from build123d import *

# Parameters (mm, degrees)
SKETCH1_R           = 1.5
BOSS_EXTRUDE1_DEPTH = 3
FILLET1_R           = 2


with BuildPart() as part:
    # Sketch1 → Boss-Extrude1 (new body)
    with BuildSketch(Plane.XY):
        with BuildLine():
            Line((-4.472135955, 4), (-12, 4))
            Line((-12, 4), (-12, -4))
            Line((-12, -4), (-4.472135955, -4))
            ThreePointArc((-4.472135955, -4), (6, 0), (-4.472135955, 4))
        make_face()
        Circle(SKETCH1_R, mode=Mode.SUBTRACT)
    extrude(amount=BOSS_EXTRUDE1_DEPTH)

    # Fillet1
    fillet1_edges = [part.edges().sort_by_distance(p)[0] for p in [
        (-4.472135955, -4, 1.5),
        (-12, -4, 1.5),
        (-12, 4, 1.5),
        (-4.472135955, 4, 1.5),
    ]]
    fillet(fillet1_edges, radius=FILLET1_R)


solid = part.part
Input: part model. Units: mm. Frame: model coordinates. Give positions to 0.01 mm unless a question says otherwise; leave off trailing zeros. Write each loop counter-clockwise with the first axis right and the second up, starting at its lowest first coordinate (ties: lowest second). Pieces come first, ordered by that corner, then holes. Notation, with made-up numbers: (-40, -39) -> (-13, -39) arc R23 ccw to (-13, -2) -> close; hole circle Ø8 at (12, 68). An arc over 180 degrees is marked (long way). Use one line per item in the form item = value. Start each with the question number.
1) Section query D-D on x = -8. Return the cut outline in (y, z), then the cut area to 3 significant figures.
2) Pin query (flat end, axial travel): pin 1 (1 mm diameter, centred on y = -1.5, z = 1, fed in from +X); pin 2 (0.9 mm diameter, centred on x = -7.5, z = 1, fed in from -Y). Return the tip coordinate at first contact, or that it passes through.
3) Section query B-B on y = 0. Return the cut outline in (x, z), then the cut area to 3 significant figures.
4) Section query A-A on z = 1.6. Return the cut outline in (x, y).
5) Section query C-C on x = 0. Return the cut outline in (y, z).
6) Draft query along Y for faces 1 (the flat face through (-8, -4, 1)), 2 (the cylindrical face through (-1.5, 0.07, 1.48)), 3 (the flat face through (-8, 4, 1)), 4 (the flat face through (-12, 0, 1)). Return one class per face: pulls with the +Y half, pulls with the -Y half, needs draft (parallel to the pull), parting line crosses it, or undercut.
7) Ray query, probe 1 along Y at (x, z) = (0, 1.7); probe 2 along X at (y, z) = (-1, 2.65); probe 3 along Y at (x, z) = (-6, 1.35). Return the intervals inside material, ascending. Write a range as from..to.
Outcome:
q1.outline = (-4, 0) -> (4, 0) -> (4, 3) -> (-4, 3) -> close
q1.area = 24.0 mm^2
q2.pin_1 = 5.92
q2.pin_2 = -4
q3.outline = (-12, 0) -> (-1.5, 0) -> (-1.5, 3) -> (-12, 3) -> close; (1.5, 0) -> (6, 0) -> (6, 3) -> (1.5, 3) -> close
q3.area = 45.0 mm^2
q4.outline = (-12, -2) arc R2 ccw to (-10, -4) -> (-5.29, -4) arc R2 cw to (-3.97, -4.5) arc R6 ccw (long way) to (-3.97, 4.5) arc R2 cw to (-5.29, 4) -> (-10, 4) arc R2 ccw to (-12, 2) -> close; hole circle Ø3 at (0, 0)
q5.outline = (-6, 0) -> (-1.5, 0) -> (-1.5, 3) -> (-6, 3) -> close; (1.5, 0) -> (6, 0) -> (6, 3) -> (1.5, 3) -> close
q6.face_1 = pulls with the -Y half
q6.face_2 = undercut
q6.face_3 = pulls with the +Y half
q6.face_4 = needs draft
q7.probe_1 = -6..-1.5, 1.5..6
q7.probe_2 = -12..-1.12, 1.12..5.92
q7.probe_3 = -4..4
